```python
from build123d import *

# Parameters (mm, degrees)
F0_W      = 32.8124985099
F0_H      = 32.8125022352
F1_DEPTH  = 84.1
F2_R      = 18.0617046785
F3_DEPTH  = 25
F4_R      = 12.861682219
F5_DEPTH  = 83.9
F6_R      = 12.5847574658
F7_DEPTH  = 95.8
F9_DEPTH  = 47.1
F10_R     = 8.1119683514
F11_DEPTH = 55.8
F12_W     = 9.392676875
F12_H     = 21.1881324649
F13_DEPTH = 42.9


with BuildPart() as f1:
    # F0 (on Top) → F1 (new body)
    with BuildSketch(Plane.XY):
        with Locations((16.4062492549, 16.4062511176)):
            Rectangle(F0_W, F0_H)
    extrude(amount=F1_DEPTH)

    # F2 (on Front) → F3 (cut)
    with BuildSketch(Plane.XZ):
        with Locations((-41.3749553263, 38.6410132051)):
            Circle(F2_R)
    extrude(amount=-F3_DEPTH, mode=Mode.SUBTRACT)

    # F4 (on face) → F5 (cut)
    with BuildSketch(Plane(origin=(0, 0, 0), x_dir=(1, 0, 0), z_dir=(0, 0, -1))):
        with Locations((16.6250001639, -16.4062511176)):
            Circle(F4_R)
    extrude(amount=-F5_DEPTH, mode=Mode.SUBTRACT)

    # F6 (on face) → F7 (cut)
    with BuildSketch(Plane(origin=(0, 0, 83.9), x_dir=(1, 0, 0), z_dir=(0, 0, -1))):
        with Locations((16.6250001639, -16.4062511176)):
            Circle(F6_R)
    extrude(amount=F7_DEPTH, mode=Mode.SUBTRACT)

    # F8 (on face) → F9 (cut)
    with BuildSketch(Plane.YZ.offset(32.8124985099)):
        Polygon((30.0061684702, 57.1961463892), (5.7924445118, 42.8192554511), (30.3500592709, 29.0380008519), align=None)
    extrude(amount=-F9_DEPTH, mode=Mode.SUBTRACT)

    # F10 (on face) → F11 (cut)
    with BuildSketch(Plane(origin=(0, 0, 0), x_dir=(0, -1, 0), z_dir=(-1, 0, 0))):
        with Locations((-18.0712518913, 14.5746218041)):
            Circle(F10_R)
    extrude(amount=-F11_DEPTH, mode=Mode.SUBTRACT)

    # F12 (on face) → F13 (cut)
    with BuildSketch(Plane(origin=(0, 0, 0), x_dir=(0, -1, 0), z_dir=(-1, 0, 0))):
        with Locations((-13.8582708314, 66.2343464792)):
            Rectangle(F12_W, F12_H)
    extrude(amount=-F13_DEPTH, mode=Mode.SUBTRACT)


solid = f1.part
```
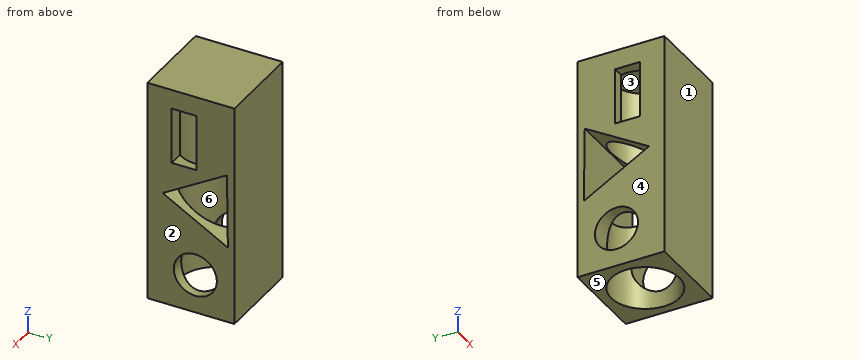
Here's how the part is built. I have some questions about the finished solid (model axes, mm). Face numbers are marked on the shaded views. A direction names the side the tool comes from. Coordinates: 2 decimals unless noted, no trailing zeros. Order: outer loops, then holes, each group sorted by start corner. A loop starts at its lowest first (then second) coordinate and runs counter-clockwise, first axis right, second up.
1) Imagine slicing it at C-C on y = 8. List the corners of the cut face in (x, z) for me, and give its area (3 significant figures).
2) I need wall thicknesses on line 1 (Y direction, x = 3, z = 57.5); line 2 (Z direction, x = 2, y = 13.5); line 3 (Z direction, x = 29.5, y = 14.5). Which ranges of each line are inside material? Lowest first, please.
3) Imagine slicing it at D-D on x = 22. List the corners of the cut face in (y, z) for me, and give its area (3 significant figures).
4) Imagine slicing it at B-B on y = 14.5. State how many separate pieces and enclosed holes the cut face has, and give its area (3 significant figures).
5) We'd pull the mould along X, two halves only. Please class the marked faces 1, 2, 3 and 4: +X half, -X half, draft (parallel to the pull), parting line (faces both ways), or undercut.
6) Will this pin go through, and if not, where does the flat tip stop? pin 1 (7.5 mm diameter, centred on x = 10.5, y = 22.5, fed in from -Z).
7) Imagine slicing it at A-A on z = 65. List the corners of the cut face in (x, y) for me (1 decimal).
8) Which directions (+Z, -Z, +X, -X, +Y, -Y) give clear straight access to the entire face, cutting with the end or side of a thin tool? Please do the marked faces 5 and 6.
Response values:
1. outline: (0, 0) - (6.89, 0) - (6.89, 41.58) - (0, 41.58) - close; (0, 44.13) - (6.89, 44.13) - (6.89, 83.9) - (26.36, 83.9) - (26.36, 44.13) - (32.81, 44.13) - (32.81, 84.1) - (0, 84.1) - close; (26.36, 0) - (32.81, 0) - (32.81, 41.58) - (26.36, 41.58) - close
1. area: 1,090 mm2
2. line 1: y = 0 to 9.16, 18.55 to 32.81
2. line 2: z = 0 to 7.87, 21.28 to 38.49, 47.4 to 55.64, 76.83 to 84.1
2. line 3: z = 0 to 7.29, 21.86 to 37.93, 47.99 to 55.64, 76.83 to 84.1
3. outline: (0, 0) - (4.72, 0) - (4.72, 83.9) - (28.09, 83.9) - (28.09, 56.06) - (30.01, 57.2) - (30.35, 29.04) - (28.09, 30.31) - (28.09, 0) - (32.81, 0) - (32.81, 84.1) - (0, 84.1) - close
3. area: 743 mm2
4. separate pieces: 7
4. enclosed holes: 0
4. area: 287 mm2
5. face 1: draft
5. face 2: +X half
5. face 3: undercut
5. face 4: -X half
6. pin 1: stops at z = 83.9
7. outline: (0, 0) - (32.8, 0) - (32.8, 9.2) - (27.3, 9.2) arc R12.9 cw to (6, 9.2) - (0, 9.2) - close; (0, 18.6) - (3.9, 18.6) arc R12.9 cw to (29.3, 18.6) - (32.8, 18.6) - (32.8, 32.8) - (0, 32.8) - close
8. face 5: -Z, +X, -X, +Y, -Y
8. face 6: -Z
